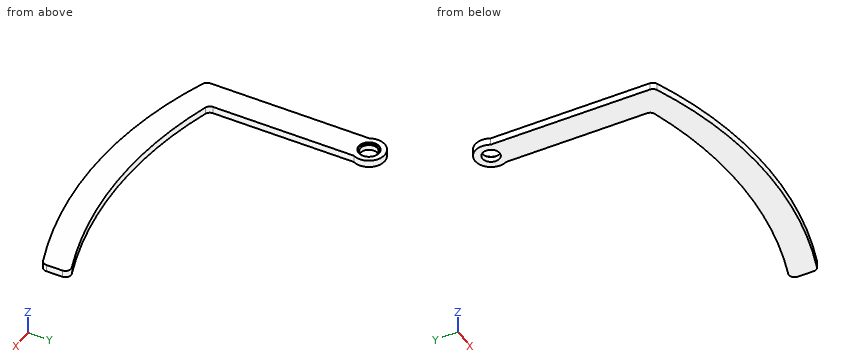
Autodesk Inventor part; units mm, degrees
ref_plane "YZ Plane" through (0, 0, 0) normal (1, 0, 0) x (0, 1, 0)
ref_plane "XZ Plane" through (0, 0, 0) normal (0, 1, 0) x (-1, 0, 0)
ref_plane "XY Plane" through (0, 0, 0) normal (0, 0, 1) x (1, 0, 0)
sketch "スケッチ1" plane through (0, 0, 0) normal (0, 0, 1) x (1, 0, 0)
  line L0 (-5, -33) -> (5, -33)
  line L1 (5, -33) -> (5, 33)
  line L2 (5, 33) -> (-5, 33)
  line L3 (-5, 33) -> (-5, -33)
  line L4 (-5, -33) -> (5, 33) construction
  line L5 (5, -33) -> (-5, 33) construction
  line L6 (-5, -33) -> (100, -33)
  line L7 (100, -33) -> (100, -23)
  line L8 (100, -23) -> (-5, -23)
  line L9 (-5, -23) -> (-5, -33)
  line L10 (47.5, -33) -> (47.5, -43)
  arc A0 (-5, -23) -> (100, -23) centre (47.5, 109.8125) ccw
  arc A1 (-5, -33) -> (100, -33) centre (47.5, 99.8125) ccw
  point P0 (0, 0)
  point P1 (5, -26.5296)
  point P2 (5, -23)
  dimension "d0" = 10
  dimension "d1" = 66
  dimension "d2" = 105
  dimension "d3" = 10
  dimension "d4" = 10
extrude "押し出し1" add sketch "スケッチ1" along normal mid plane 2.5 contours L3 A0 L1 L0 | L0 L6 L10 A1 | L1 A0 L6 | L3 L2 L1 L8 | L8 L1 A0 | L10 L6 A1 | A0 L7 L6 picked at (-0.5654, -23.4196)
sketch "スケッチ2" plane through (0, 0, 1.25) normal (0, 0, 1) x (1, 0, 0)
  line L0 (5, 33) -> (-5, 33)
  line L1 (5, -26.5296) -> (5, 33)
  circle A0 centre (0, 28) radius 3.05
  circle A1 centre (0, 28) radius 3.65
  point P0 (0, 0)
  dimension "d7" = 5
  dimension "d8" = 5
  dimension "d9" = 6.1
  dimension "d10" = 7.3
extrude "押し出し2" cut sketch "スケッチ2" against normal blind 0.6 contours A0 | A1
sketch "スケッチ3" plane through (0, 28, 0.65) normal (0, 0, 1) x (1, 0, 0)
  circle A0 centre (0, 0) radius 3.05
  point P0 (0, -28)
  dimension "d13" = 6.1
extrude "押し出し3" cut sketch "スケッチ3" against normal blind 1.9
sketch "スケッチ6" plane through (0, 0, 1.25) normal (0, 0, 1) x (1, 0, 0)
  circle A0 centre (0, 28) radius 3.65
  line L0 (-5, 33) -> (-5, -33)
  arc A1 (-5, -33) -> (100, -33) centre (47.5, 99.8125) ccw
  line L1 (100, -33) -> (100, -23)
  arc A2 (5, -26.5296) -> (100, -23) centre (47.5, 109.8125) ccw
  line L2 (5, -26.5296) -> (5, 33)
  line L3 (5, 33) -> (-5, 33)
  circle A3 centre (0, 28) radius 5.65
  point P0 (0, 0)
  point P1 (-5, 25.3689)
  point P2 (-5, 30.6311)
  point P3 (-2.6311, 33)
  point P4 (2.6311, 33)
  point P5 (5, 30.6311)
  point P6 (5, 25.3689)
  dimension "d18" = 11.3
extrude "押し出し5" add sketch "スケッチ6" against normal blind 2.5 contours L0 A3 | A3 L3 | L2 A3
sketch "スケッチ7" plane through (0, 0, 1.25) normal (0, 0, 1) x (1, 0, 0)
  circle A0 centre (0, 28) radius 3.65
  line L0 (-5, 33) -> (-5, 30.6311)
  arc A1 (-5, 30.6311) -> (-5, 25.3689) centre (0, 28) ccw
  line L1 (-5, 25.3689) -> (-5, -33)
  arc A2 (-5, -33) -> (100, -33) centre (47.5, 99.8125) ccw
  line L2 (100, -33) -> (100, -23)
  arc A3 (5, -26.5296) -> (100, -23) centre (47.5, 109.8125) ccw
  line L3 (5, -26.5296) -> (5, 25.3689)
  arc A4 (5, 25.3689) -> (5, 30.6311) centre (0, 28) ccw
  line L4 (5, 30.6311) -> (5, 33)
  line L5 (5, 33) -> (2.6311, 33)
  arc A5 (2.6311, 33) -> (-2.6311, 33) centre (0, 28) ccw
  line L6 (-2.6311, 33) -> (-5, 33)
  circle A6 centre (0, 28) radius 5.65
  point P0 (0, 0)
  point P1 (-2.6311, 33)
  point P2 (2.6311, 33)
extrude "押し出し6" cut sketch "スケッチ7" against normal blind 2.5 contours L6 A6 L0 | L5 L4 A6
fillet "フィレット1" radius 2 4 edges at (-5, -33, 0) (5, -26.5296, 0) (100, -23, 0) (100, -33, 0)
properties part number "指_小"
The model under review builds one solid part; all positions refer to its coordinate system, in mm. Round coordinates to 2 decimals unless told otherwise and drop trailing zeros. Loops run counter-clockwise (first coordinate to the right, second up) from the corner with the lowest first, then second, coordinate; pieces in that order, holes last. Notation, with made-up numbers: (68.25, 54.25) -> (96.25, 54.25) arc R26 ccw to (96.25, 83.25) -> close; hole circle Ø11 at (3, 53.25). An arc over 180 degrees is marked (long way). Answer in a Markdown table with one row per item.
1) Wall thickness on line 1 along X through (y, z) = (1, 1); line 2 along Y through (x, z) = (0, 0.8); line 3 along Y through (x, z) = (0, -0.55): over which ranges is each line inside the solid? List them lowest first.
Taken from the geometry:
| item | result |
|---|---|
| line 1 | x = -5 to 5 |
| line 2 | y = -34.87 to 24.35, 31.65 to 33.65 |
| line 3 | y = -34.87 to 24.95, 31.05 to 33.65 |
2) Consider section A-A, the plane y = 28. Write out the cut boundary in (x, z), plus the area to 3 significant figures.
Taken from the geometry:
| item | result |
|---|---|
| outline | (-5.65, -1.25) -> (-3.05, -1.25) -> (-3.05, 0.65) -> (-3.65, 0.65) -> (-3.65, 1.25) -> (-5.65, 1.25) -> close; (3.05, -1.25) -> (5.65, -1.25) -> (5.65, 1.25) -> (3.65, 1.25) -> (3.65, 0.65) -> (3.05, 0.65) -> close |
| area | 12.3 mm² |
3) Consider section C-C, the plane x = 0. Write out the cut boundary in (y, z).
Taken from the geometry:
| item | result |
|---|---|
| outline | (-34.87, -1.25) -> (24.95, -1.25) -> (24.95, 0.65) -> (24.35, 0.65) -> (24.35, 1.25) -> (-34.87, 1.25) -> close; (31.05, -1.25) -> (33.65, -1.25) -> (33.65, 1.25) -> (31.65, 1.25) -> (31.65, 0.65) -> (31.05, 0.65) -> close |
4) For pin 1 Ø4.5 at (x, y) = (0, 28) entering from +Z; pin 2 Ø0.8 at (y, z) = (-10, 0.5) entering from -X; pin 3 Ø0.8 at (y, z) = (1, 0) entering from +X, all flat-tipped, find the tip position at first contact; note any pin that passes through.
Taken from the geometry:
| item | result |
|---|---|
| pin 1 | passes through |
| pin 2 | stops at x = -5 |
| pin 3 | stops at x = 5 |
5) Consider section D-D, the plane y = -29.5. Write out the cut boundary in (x, z).
Taken from the geometry:
| item | result |
|---|---|
| outline | (-5, -1.25) -> (16.08, -1.25) -> (16.08, 1.25) -> (-5, 1.25) -> close; (78.92, -1.25) -> (100, -1.25) -> (100, 1.25) -> (78.92, 1.25) -> close |
